from build123d import *

# Parameters (mm, degrees)
FILLET1_R      = 2.54
CHAMFER1_SIZE  = 2.54
CHAMFER1_SIZE2 = 2.60331341


with BuildPart() as part:
    # Sketch1 → Revolve1 (revolve)
    with BuildSketch(Plane.XY, mode=Mode.PRIVATE) as revolve1_sk:
        Polygon((0, 0), (0, 7.493), (66.04, 9.0805), (71.12, 9.0805), (82.562216058, 79.375), (87.642216058, 79.375), (104.14, 69.85), (104.14, 0), align=None)
    revolve(revolve1_sk.sketch.rotate(Axis((-13.738402674, 0, 0), (1, 0, 0)), 90), axis=Axis((-13.738402674, 0, 0), (1, 0, 0)))

    # Fillet1
    fillet1_edges = [part.edges().sort_by_distance(p)[0] for p in [
        (71.12, 0, -9.0805),
    ]]
    fillet(fillet1_edges, radius=FILLET1_R)

    # Chamfer1
    chamfer1_edges = [part.edges().sort_by_distance(p)[0] for p in [
        (0, 0, -7.493),
    ]]
    chamfer1_side = [part.faces().sort_by_distance(p)[0] for p in [
        (33.02, 0, -8.28675),
    ]]
    chamfer(chamfer1_edges, length=CHAMFER1_SIZE, length2=CHAMFER1_SIZE2, reference=chamfer1_side[0])


solid = part.part
Can you work these out from the model? Positions are in its coordinate system, mm. A direction names the side the tool comes from. Give positions to 0.01 mm unless a question says otherwise; leave off trailing zeros. Write each loop counter-clockwise with the first axis right and the second up, starting at its lowest first coordinate (ties: lowest second). Pieces come first, ordered by that corner, then holes. Notation, with made-up numbers: M -35,1.5 L -18,1.5 A18 cw -18,26.5 Z; hole C -16.75,85.25 d8. An arc over 180 degrees is marked long. Answer in a Markdown table with one row per item. Add a question column.
Item 1: Imagine slicing it at A-A, the plane x = 19. Write out the boundary of the cut face in (y, z).
Item 2: Please list where these lines run through material, in increasing order: L1, parallel to X at y = 64, z = -14; L2, parallel to Z at x = 90.5, y = 53; L3, parallel to X at y = -46.5, z = 28.5.
Item 3: For pin 1 Ø6 at (y, z) = (-16, -51) entering from -X; pin 2 Ø6 at (x, z) = (84.5, 25.5) entering from +Y; pin 3 Ø5 at (y, z) = (-46, -52.5) entering from -X, each with a flat end and sliding along its axis, tell me the tip position at first contact or that it passes through.
Item 4: On a 3-axis mill with a long thin cutter (end or side, diameter ignored), from which of +Z, -Z, +X, -X, +Y, -Y can I reach the whole of each face in a straight line? I mean faces 1 (the cylindrical face through (85.14, -23.84, 75.71)), 2 (the conical face through (34.73, 7.39, 3.84)). Say none if no direction works.
Item 5: Imagine slicing it at B-B, the plane x = 76. Write out the boundary of the cut face in (y, z).
Evaluation:
| question | item | result |
|---|---|---|
| 1 | outline | C 0,0 d15.9 |
| 2 | L1 | x = 80.31 to 104.14 |
| 2 | L2 | z = -56.85 to 56.85 |
| 2 | L3 | x = 78.52 to 104.14 |
| 3 | pin 1 | stops at x = 77.85 |
| 3 | pin 2 | stops at y = 76.12 |
| 3 | pin 3 | stops at x = 80.6 |
| 4 | face 1 | +X, -X |
| 4 | face 2 | -X |
| 5 | outline | C 0,0 d78.12 |
